Check sheet for the modelled part. Datum: model origin and axes. Units: mm. A direction names the side the tool comes from. Round coordinates to 2 decimals unless told otherwise and drop trailing zeros. Loops run counter-clockwise (first coordinate to the right, second up) from the corner with the lowest first, then second, coordinate; pieces in that order, holes last. Notation, with made-up numbers: (-11, -12.5) -> (37, -12.5) arc R26 cw to (37, 1.5) -> close; hole circle Ø1 at (-21, -12). An arc over 180 degrees is marked (long way). Return JSON: item names as keys, results as strings.
from build123d import *

# Parameters (mm, degrees)
BOSS_EXTRUDE1_DEPTH = 1.5875
SKETCH3_R           = 1.63195
CUT_EXTRUDE1_DEPTH  = 95.855674265


with BuildPart() as part:
    # Sketch1 → Boss-Extrude1 (new body)
    with BuildSketch(Plane.XY):
        with BuildLine():
            Line((0, 47.625), (0, 18.415))
            Line((0, 18.415), (2.921, 18.415))
            ThreePointArc((2.921, 18.415), (7.411128061, 16.555128061), (9.271, 12.065))
            Line((9.271, 12.065), (9.271, 0))
            Line((9.271, 0), (58.801, 0))
            Line((58.801, 0), (58.801, 12.065))
            ThreePointArc((58.801, 12.065), (60.660871939, 16.555128061), (65.151, 18.415))
            Line((65.151, 18.415), (68.072, 18.415))
            Line((68.072, 18.415), (68.072, 47.625))
            Line((68.072, 47.625), (65.151, 47.625))
            ThreePointArc((65.151, 47.625), (60.660871939, 49.484871939), (58.801, 53.975))
            Line((58.801, 53.975), (58.801, 66.04))
            Line((58.801, 66.04), (9.271, 66.04))
            Line((9.271, 66.04), (9.271, 53.975))
            ThreePointArc((9.271, 53.975), (7.411128061, 49.484871939), (2.921, 47.625))
            Line((2.921, 47.625), (0, 47.625))
        make_face()
    extrude(amount=BOSS_EXTRUDE1_DEPTH)

    # Sketch3 → Cut-Extrude1 (cut, through all)
    with BuildSketch(Plane.XY.offset(1.5875)):
        with Locations((54.991, 62.23)):
            Circle(SKETCH3_R)
        with Locations((54.991, 3.81)):
            Circle(SKETCH3_R)
        with Locations((13.081, 3.81)):
            Circle(SKETCH3_R)
        with Locations((13.081, 62.23)):
            Circle(SKETCH3_R)
    extrude(amount=-CUT_EXTRUDE1_DEPTH, mode=Mode.SUBTRACT)


solid = part.part
Q1. Material ranges on line 1 (Y direction, x = 65.5, z = 1.45) (3 decimals); line 2 (X direction, y = 3, z = 0.25); line 3 (Y direction, x = 55.5, z = 1.45), recorded low to high.
Results list:
{"line 1": "18.415 to 47.625", "line 2": "9.27 to 11.66, 14.5 to 53.57, 56.41 to 58.8", "line 3": "0 to 2.26, 5.36 to 60.68, 63.78 to 66.04"}
Q2. Tool access check on faces 4 (the flat face through (1, 47.625, 1)), 5 (the flat face through (58.801, 60, 1)), 6 (the flat face through (34, 33, 1.588)). Record the directions out of +Z, -Z, +X, -X, +Y, -Y that give a thin tool (end or side, any length) a straight path to the whole face; none if there is none.
Results list:
{"face 4": "+Z, -Z, -X, +Y", "face 5": "+Z, -Z, +X, +Y", "face 6": "+Z, +X, -X, +Y, -Y"}
Q3. Section check A-A (y = 3.81). Record the boundary of the cut face in (x, z), then the cut area to 3 significant figures.
Results list:
{"outline": "(9.27, 0) -> (11.45, 0) -> (11.45, 1.59) -> (9.27, 1.59) -> close; (14.71, 0) -> (53.36, 0) -> (53.36, 1.59) -> (14.71, 1.59) -> close; (56.62, 0) -> (58.8, 0) -> (58.8, 1.59) -> (56.62, 1.59) -> close", "area": "68.3 mm^2"}
Q4. Go/stop test with flat-tipped pins: pin 1 (0.8 mm diameter, centred on x = 66, z = 0.5, fed in from +Y) (3 decimals); pin 2 (0.5 mm diameter, centred on y = 63, z = 1, fed in from -X); pin 3 (0.8 mm diameter, centred on y = 58, z = 1, fed in from +X); pin 4 (2.5 mm diameter, centred on x = 54.991, y = 62.23, fed in from +Z). Record where each tip stops, or that it passes through.
Results list:
{"pin 1": "y = 47.625", "pin 2": "x = 9.27", "pin 3": "x = 58.8", "pin 4": "through"}
Q5. Section check B-B (z = 1.15). Record the boundary of the cut face in (x, y) (3 decimals), then the cut area to 3 significant figures.
Results list:
{"outline": "(0, 18.415) -> (2.921, 18.415) arc R6.35 cw to (9.271, 12.065) -> (9.271, 0) -> (58.801, 0) -> (58.801, 12.065) arc R6.35 cw to (65.151, 18.415) -> (68.072, 18.415) -> (68.072, 47.625) -> (65.151, 47.625) arc R6.35 cw to (58.801, 53.975) -> (58.801, 66.04) -> (9.271, 66.04) -> (9.271, 53.975) arc R6.35 cw to (2.921, 47.625) -> (0, 47.625) -> close; hole circle Ø3.264 at (13.081, 3.81); hole circle Ø3.264 at (13.081, 62.23); hole circle Ø3.264 at (54.991, 3.81); hole circle Ø3.264 at (54.991, 62.23)", "area": "3,810 mm^2"}
Q6. Draft check along X on faces 1 (the flat face through (1, 18.415, 1)), 2 (the flat face through (9.271, 6, 1)), 3 (the cylindrical face through (53.788, 63.333, 0.805)). Enter one of: released by +X, released by -X, zero draft, split by the parting line, or undercut.
Results list:
{"face 1": "zero draft", "face 2": "released by -X", "face 3": "undercut"}
